The model under review builds one solid part; all positions refer to its coordinate system, in mm. Round coordinates to 2 decimals unless told otherwise and drop trailing zeros. Order: outer loops, then holes, each group sorted by start corner. A loop starts at its lowest first (then second) coordinate and runs counter-clockwise, first axis right, second up. Notation, with made-up numbers: (73, 31.5) -> (112, 31.5) arc R10 cw to (112, 39.5) -> close; hole circle Ø8 at (-29.5, 27.25). An arc over 180 degrees is marked (long way). Return JSON: item names as keys, results as strings. Group by question number.
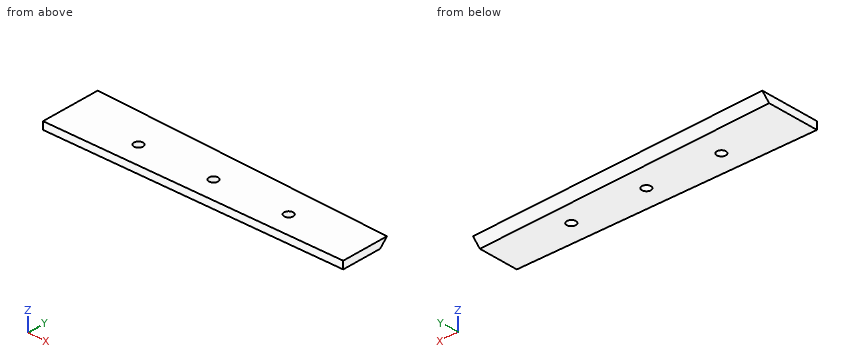
from build123d import *

# Parameters (mm, degrees)
SKETCH1_W           = 5
SKETCH1_H           = 40
BOSS_EXTRUDE1_DEPTH = 200
CUT_EXTRUDE2_DEPTH  = 5
CHAMFER1_SIZE       = 5
SKETCH2_R           = 3
CUT_EXTRUDE1_DEPTH  = 5
LPATTERN1_COUNT     = 3
LPATTERN1_PITCH     = 50


with BuildPart() as part:
    # Sketch1 → Boss-Extrude1 (new body)
    with BuildSketch(Plane(origin=(0, 0, 0), x_dir=(0, 0, -1), z_dir=(1, 0, 0))):
        with Locations((418.326871087, -169.232517464)):
            Rectangle(SKETCH1_W, SKETCH1_H)
    extrude(amount=BOSS_EXTRUDE1_DEPTH)

    # Sketch3 → Cut-Extrude2 (cut)
    with BuildSketch(Plane.XY.offset(-415.826871087)):
        Polygon((0, -149.232517464), (200, -149.232517464), (200, -157.232517464), align=None)
    extrude(amount=-CUT_EXTRUDE2_DEPTH, mode=Mode.SUBTRACT)

    # Chamfer1
    chamfer1_edges = [part.edges().sort_by_distance(p)[0] for p in [
        (100, -153.232517464, -420.826871087),
    ]]
    chamfer(chamfer1_edges, length=CHAMFER1_SIZE - 0.0001)  # a hair under: the kernel refuses the full size

    # Sketch2 → Cut-Extrude1 (cut)
    with BuildSketch(Plane(origin=(0, 0, -420.826871087), x_dir=(-1, 0, 0), z_dir=(0, 0, -1))):
        with Locations((-50, -174.232517464)):
            Circle(SKETCH2_R)
    cut_extrude1 = extrude(amount=-CUT_EXTRUDE1_DEPTH, mode=Mode.SUBTRACT)

    # LPattern1: Cut-Extrude1 ×3
    with Locations(*[(i * LPATTERN1_PITCH, 0, 0) for i in range(1, LPATTERN1_COUNT)]):
        add(cut_extrude1, mode=Mode.SUBTRACT)


solid = part.part
Item 1: Wall thickness on line 1 along X through (y, z) = (-173.5, -418.9); line 2 along X through (y, z) = (-172.5, -416.5); line 3 along Y through (x, z) = (100, -417.8): over which ranges is each line inside the solid? List them lowest first.
Item 2: Insertion check: pin 1 Ø2 at (x, z) = (88, -418.5) entering from +Y; pin 2 Ø5.5 at (x, y) = (150, -174.23) entering from -Z. Each pin has a flat end and moves straight along its axis. Give the tip position at first contact, or say it passes through.
Item 3: Consider section B-B on z = -420.05. State the section outline as (x, y) points, plus the area to 3 significant figures.
Values:
{
 "1": {"line 1": "0 to 47.09, 52.91 to 97.09, 102.91 to 147.09, 152.91 to 200", "line 2": "0 to 47.55, 52.45 to 97.55, 102.45 to 147.55, 152.45 to 200", "line 3": "-189.23 to -177.23, -171.23 to -155.21"},
 "2": {"pin 1": "y = -154.43", "pin 2": "through"},
 "3": {"outline": "(0, -189.23) -> (200, -189.23) -> (200, -161.46) -> (0, -153.46) -> close; hole circle Ø6 at (50, -174.23); hole circle Ø6 at (100, -174.23); hole circle Ø6 at (150, -174.23)", "area": "6,270 mm^2"}
}
